from build123d import *

# Parameters (mm, degrees)
SKETCH_1_R      = 2.25
EXTRUDE_1_DEPTH = 2.5
FILLET_1_R      = 0.5


with BuildPart() as part:
    # Эскиз1 → Бобышка-Вытянуть1 (new body)
    with BuildSketch(Plane(origin=(0, 0, 0), x_dir=(0, 0, -1), z_dir=(1, 0, 0))):
        with BuildLine():
            ThreePointArc((22.943818195, 7.757072943), (20.83949046, 10.565703525), (17.340266807, 10.834096505))
            Line((17.340266807, 10.834096505), (7.414281192, 7.221333195))
            ThreePointArc((7.414281192, 7.221333195), (-0.89095562, 4.985699873), (-9.456459328, 4.206494465))
            Line((-9.456459328, 4.206494465), (-252.5, 3.087186175))
            Line((-252.5, 3.087186175), (-252.5, 7))
            Line((-252.5, 7), (-257.5, 7))
            Line((-257.5, 7), (-257.5, 3.064159266))
            Line((-257.5, 3.064159266), (-262.5, 3.041132357))
            Line((-262.5, 3.041132357), (-262.5, 7))
            Line((-262.5, 7), (-267.5, 7))
            Line((-267.5, 7), (-267.5, 3.018105448))
            Line((-267.5, 3.018105448), (-380, 2.5))
            ThreePointArc((-380, 2.5), (-382.5, 0), (-380, -2.5))
            Line((-380, -2.5), (-0.019572665, -4.24995493))
            ThreePointArc((-0.019572665, -4.24995493), (1.046958504, -4.119026328), (2.046563679, -3.724792223))
            Line((2.046563679, -3.724792223), (22.943818195, 7.757072943))
        make_face()
        with BuildLine():
            Line((18.793852416, 6.840402867), (18.161115151, 8.578834215))
            ThreePointArc((18.161115151, 8.578834215), (19.5756962, 8.517072273), (20.532283764, 7.473140132))
            Line((20.532283764, 7.473140132), (18.793852416, 6.840402867))
        make_face(mode=Mode.SUBTRACT)
        Circle(SKETCH_1_R, mode=Mode.SUBTRACT)
    extrude(amount=EXTRUDE_1_DEPTH)

    # Скругление1
    fillet_1_edges = [part.edges().sort_by_distance(p)[0] for p in [
        (2.5, 0, 2.25),
        (2.5, 7.156771499, -19.66306809),
        (2.5, 7.709618541, -18.477483783),
        (0, 0, 2.25),
        (0, 7.709618541, -18.477483783),
        (0, 7.156771499, -19.66306809),
        (0, 8.517072273, -19.5756962),
        (1.25, 7, 267.5),
        (1.25, 7, 252.5),
        (2.5, 8.517072273, -19.5756962),
    ]]
    fillet(fillet_1_edges, radius=FILLET_1_R)


solid = part.part
The listing builds one solid part. Answer for the finished solid, in the listing's coordinates (mm). Round coordinates to 2 decimals unless told otherwise and drop trailing zeros. Write each loop counter-clockwise with the first axis right and the second up, starting at its lowest first coordinate (ties: lowest second). Pieces come first, ordered by that corner, then holes. Notation, with made-up numbers: (-19.75, 13) - (0.25, 13) arc R11 cw to (0.25, 27) - close; hole circle Ø1 at (18.25, 10.5). An arc over 180 degrees is marked (long way). Use a Markdown table: item, result. Add a question column.
1. Consider line 1 (Y direction, x = 1.6, z = 315); line 2 (Y direction, x = 2.25, z = 337.5); line 3 (Y direction, x = 0.9, z = 0). Determine where each line is inside the solid, lowest interval first.
2. The part is cut by section C-C (z = 154). Write down the section's boundary in (x, y).
3. The part is cut by section B-B (z = 88.5). Write down the section's boundary in (x, y), and give its area (3 significant figures).
4. Flat-ended cylindrical pins translate along their axes: P1, Ø1.2, axis at x = 2, z = 256, coming from the +Y side; P2, Ø0.8, axis at x = 2, y = 5, coming from the +Z side; P3, Ø7, axis at y = 0, z = 0, coming from the +X side; P4, Ø1.5, axis at x = 0.5, z = 233.5, coming from the -Y side. Find the tip coordinate at first contact, or state that the pin passes through.
5. The part is cut by section A-A (x = 0.9). Write down the section's boundary in (y, z).
Reported:
| question | item | result |
|---|---|---|
| 1 | line 1 | -2.8 to 2.8 |
| 1 | line 2 | -2.7 to 2.7 |
| 1 | line 3 | -4.25 to -2.25, 2.25 to 5.15 |
| 2 | outline | (0, -3.54) - (2.5, -3.54) - (2.5, 3.54) - (0, 3.54) - close |
| 3 | outline | (0, -3.84) - (2.5, -3.84) - (2.5, 3.84) - (0, 3.84) - close |
| 3 | area | 19.2 mm^2 |
| 4 | P1 | y = 7 |
| 4 | P2 | z = 267.5 |
| 4 | P3 | x = 2.5 |
| 4 | P4 | y = -3.18 |
| 5 | outline | (-4.25, 0.02) arc R4.25 ccw to (-3.72, -2.05) - (7.76, -22.94) arc R4.25 ccw to (10.83, -17.34) - (7.22, -7.41) arc R50 cw to (4.21, 9.46) - (3.09, 252.5) - (6.5, 252.5) arc R0.5 ccw to (7, 253) - (7, 257.5) - (3.06, 257.5) - (3.04, 262.5) - (7, 262.5) - (7, 267) arc R0.5 ccw to (6.5, 267.5) - (3.02, 267.5) - (2.5, 380) arc R2.5 ccw to (-2.5, 380) - close; hole circle Ø4.5 at (0, 0); hole (6.84, -18.79) - (7.47, -20.53) arc R1.85 ccw to (8.58, -18.16) - close |
